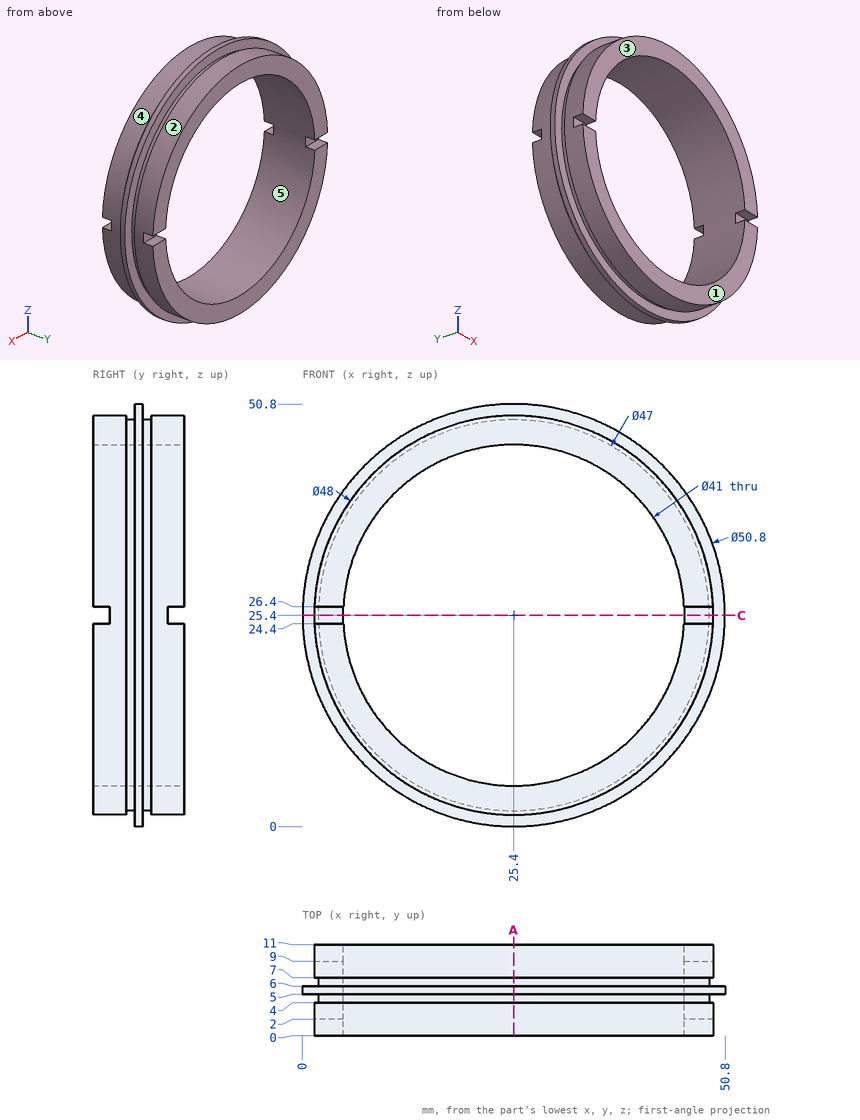
Geometry check sheet. Reference: drawing and pictorial views, mm from the part's lowest x, y, z. A direction names the side the tool comes from. Coordinates: 2 decimals unless noted, no trailing zeros. Write each loop counter-clockwise with the first axis right and the second up, starting at its lowest first coordinate (ties: lowest second). Pieces come first, ordered by that corner, then holes. Notation, with made-up numbers: M 76,3 L 116,3 A27 ccw 116,35 Z; hole C -1,-40 d8. An arc over 180 degrees is marked long. Write item = value, one per line. Start each with the question number.
1. Sectioned sample at C-C (z = 25.4). Record the cut outline in (x, y).
2. Tool access check on the marked faces 1 and 2. Record the directions out of +Z, -Z, +X, -X, +Y, -Y that give a thin tool (end or side, any length) a straight path to the whole face; none if there is none.
3. Thickness scan on probe 1 along X at (y, z) = (3.75, 25.4); probe 2 along X at (y, z) = (4.5, 25.4); probe 3 along Z at (x, y) = (17, 1). Record the ranges inside material, lowest first.
4. Sectioned sample at A-A (x = 25.4). Record the cut outline in (y, z), then the cut area to 3 significant figures.
5. Mould release check, pull along X, two halves, no side actions. Record for the marked faces 3, 4 and 5: pulls with the +X half, pulls with the -X half, needs draft (parallel to the pull), parting line crosses it, or undercut.
6. Go/stop test with flat-tipped pins: pin 1 (1.6 mm diameter, centred on x = 3, y = 1, fed in from -Z); pin 2 (0.6 mm diameter, centred on x = 47, y = 1, fed in from -Z); pin 3 (1 mm diameter, centred on x = 3, z = 25.5, fed in from -Y). Record where each tip stops, or that it passes through.
The answers:
q1.outline = M 0,5 L 1.9,5 L 1.9,4 L 1.4,4 L 1.4,2 L 4.9,2 L 4.9,9 L 1.4,9 L 1.4,7 L 1.9,7 L 1.9,6 L 0,6 Z; M 45.9,2 L 49.4,2 L 49.4,4 L 48.9,4 L 48.9,5 L 50.8,5 L 50.8,6 L 48.9,6 L 48.9,7 L 49.4,7 L 49.4,9 L 45.9,9 Z
q2.face_1 = +Z, -Z, +X, -X, -Y
q2.face_2 = +Y
q3.probe_1 = 1.4 to 4.9, 45.9 to 49.4
q3.probe_2 = 1.9 to 4.9, 45.9 to 48.9
q3.probe_3 = 2.92 to 6.7, 44.1 to 47.88
q4.outline = M 0,1.4 L 4,1.4 L 4,1.9 L 5,1.9 L 5,0 L 6,0 L 6,1.9 L 7,1.9 L 7,1.4 L 11,1.4 L 11,4.9 L 0,4.9 Z; M 0,45.9 L 11,45.9 L 11,49.4 L 7,49.4 L 7,48.9 L 6,48.9 L 6,50.8 L 5,50.8 L 5,48.9 L 4,48.9 L 4,49.4 L 0,49.4 Z
q4.area = 77.8 mm²
q5.face_3 = needs draft
q5.face_4 = parting line crosses it
q5.face_5 = undercut
q6.pin_1 = 14.94
q6.pin_2 = 14.34
q6.pin_3 = 2
